The listing builds one solid part. Answer for the finished solid, in the listing's coordinates (mm). A direction names the side the tool comes from. Coordinates: 2 decimals unless noted, no trailing zeros. Write each loop counter-clockwise with the first axis right and the second up, starting at its lowest first coordinate (ties: lowest second). Pieces come first, ordered by that corner, then holes.
(1) For a pull along Y with two mould halves and no side action, classify faces 1 (the cylindrical face through (7.907, 10.744, 0.178)), 2 (the flat face through (10.319, 1, 0)), 3 (the cylindrical face through (7.99, 11.76, 0.18)) as +Y half, -Y half, draft (parallel to the pull), parting line (faces both ways), or undercut.
(2) The part is cut by section A-A on y = 8. Determine the outline of the cut face in (x, z).
(3) The part is cut by section C-C on z = -7. Determine the outline of the cut face in (x, y).
(4) Given P1, Ø1.5, axis at x = 7, z = 3.5, coming from the +Y side, flat-ended and moving along its own axis, determine where the tip first touches the part or whether it passes through.
(5) Straight lines are drawn through the part: line 1 (X direction, y = -1.5, z = 9.75); line 2 (Y direction, x = -1.5, z = -10); line 3 (Y direction, x = -7, z = 2.75). For each, find the intervals that lie inside material, in ascending order.
(6) The part is cut by section D-D on x = 3. Determine the outline of the cut face in (y, z).
(7) The part is cut by section B-B on x = 7.5. Determine the outline of the cut face in (y, z).
(8) Which of the six approach directions +Z, -Z, +X, -X, +Y, -Y give full straight-line access (tool end or side, diameter ignored) to faces 4 (the flat face through (-10.319, 1, 0)), 5 (the cylindrical face through (-7.968, 10.744, 0.178))?
from build123d import *

# Parameters (mm, degrees)
BASE_EXTRUDE_DEPTH = 12.7


with BuildPart() as part:
    # Sketch1 → Base-Extrude (new, symmetric)
    with BuildSketch(Plane.XY):
        with BuildLine():
            Line((-10.31875, 9.37895), (-10.31875, -7.874))
            ThreePointArc((-10.31875, -7.874), (-10.02117049, -8.59242049), (-9.30275, -8.89))
            Line((-9.30275, -8.89), (9.30275, -8.89))
            ThreePointArc((9.30275, -8.89), (10.02117049, -8.59242049), (10.31875, -7.874))
            Line((10.31875, -7.874), (10.31875, 9.37895))
            ThreePointArc((10.31875, 9.37895), (7.9375, 11.7602), (5.55625, 9.37895))
            Line((5.55625, 9.37895), (6.57225, 9.37895))
            ThreePointArc((6.57225, 9.37895), (7.9375, 10.7442), (9.30275, 9.37895))
            Line((9.30275, 9.37895), (9.30275, -7.874))
            Line((9.30275, -7.874), (-9.30275, -7.874))
            Line((-9.30275, -7.874), (-9.30275, 9.37895))
            ThreePointArc((-9.30275, 9.37895), (-7.9375, 10.7442), (-6.57225, 9.37895))
            Line((-6.57225, 9.37895), (-5.55625, 9.37895))
            ThreePointArc((-5.55625, 9.37895), (-7.9375, 11.7602), (-10.31875, 9.37895))
        make_face()
    extrude(amount=BASE_EXTRUDE_DEPTH, both=True)


solid = part.part
Model answer:
1. face 1: undercut
1. face 2: draft
1. face 3: +Y half
2. outline: (-10.32, -12.7) - (-9.3, -12.7) - (-9.3, 12.7) - (-10.32, 12.7) - close; (9.3, -12.7) - (10.32, -12.7) - (10.32, 12.7) - (9.3, 12.7) - close
3. outline: (-10.32, -7.87) arc R1.02 ccw to (-9.3, -8.89) - (9.3, -8.89) arc R1.02 ccw to (10.32, -7.87) - (10.32, 9.38) arc R2.38 ccw to (5.56, 9.38) - (6.57, 9.38) arc R1.37 cw to (9.3, 9.38) - (9.3, -7.87) - (-9.3, -7.87) - (-9.3, 9.38) arc R1.37 cw to (-6.57, 9.38) - (-5.56, 9.38) arc R2.38 ccw to (-10.32, 9.38) - close
4. P1: stops at y = 11.75
5. line 1: x = -10.32 to -9.3, 9.3 to 10.32
5. line 2: y = -8.89 to -7.87
5. line 3: y = -8.89 to -7.87, 10.37 to 11.57
6. outline: (-8.89, -12.7) - (-7.87, -12.7) - (-7.87, 12.7) - (-8.89, 12.7) - close
7. outline: (-8.89, -12.7) - (-7.87, -12.7) - (-7.87, 12.7) - (-8.89, 12.7) - close; (10.67, -12.7) - (11.72, -12.7) - (11.72, 12.7) - (10.67, 12.7) - close
8. face 4: +Z, -Z, -X, +Y, -Y
8. face 5: +Z, -Z
